Model file for the job. Use its own axes, mm. Round coordinates to 2 decimals unless told otherwise and drop trailing zeros. Loops run counter-clockwise (first coordinate to the right, second up) from the corner with the lowest first, then second, coordinate; pieces in that order, holes last. Notation, with made-up numbers: M 39,12 L 89,12 A24 ccw 89,33 Z; hole C -38.5,16 d9. An arc over 180 degrees is marked long. Use a Markdown table: item, result. Add a question column.
Q1. Pin check, flat tips, straight feed: pin 1 (5.5 mm diameter, centred on x = -31.75, y = -6.35, fed in from -Z); pin 2 (2 mm diameter, centred on x = 81.5, y = -4.5, fed in from +Z); pin 3 (6.5 mm diameter, centred on x = 82.55, y = -6.35, fed in from -Z). Stop position of each tip, or through.
Q2. Cut at A-A (z = 3.5). Give the cut face in (x, y).
Q3. Cut at D-D (x = 82.55). Give the cut face in (y, z).
Q4. Cut at B-B (x = 120.65). Give the cut face in (y, z), plus the area to 3 significant figures.
Q5. Cut at C-C (y = -6.35). State how many separate pieces and enclosed holes the cut face has, plus the area to 3 significant figures.
Q6. Probe line 1 (X direction, y = -6.35, z = 7.25); line 2 (X direction, y = -11, z = 4.5); line 3 (Y direction, x = 82.55, z = 11.5). List the from-to ranges inside material, lowest first. Write a range as from..to.
from build123d import *

# Parameters (mm, degrees)
F0_W      = 254
F0_H      = 12.7
F1_DEPTH  = 12.7
F2_W      = 12.7
F2_H      = 6.35
F3_DEPTH  = 12.701
F4_R      = 2.794
F5_DEPTH  = 6.351
F6_R      = 4.7625
F7_DEPTH  = 5.08
F8_R      = 2.794
F9_DEPTH  = 12.701
F10_R     = 4.7625
F10_R_2   = 2.794
F11_DEPTH = 5.08


with BuildPart() as f1:
    # F0 (on Top) → F1 (new body)
    with BuildSketch(Plane.XY):
        with Locations((0, -6.35)):
            Rectangle(F0_W, F0_H)
    extrude(amount=F1_DEPTH)

    # F2 (on face) → F3 (cut, through all)
    with BuildSketch(Plane.XZ.offset(12.7)):
        with Locations((82.55, 3.175)):
            Rectangle(F2_W, F2_H)
        with Locations((31.75, 3.175)):
            Rectangle(F2_W, F2_H)
        with Locations((-31.75, 3.175)):
            Rectangle(F2_W, F2_H)
        with Locations((-82.55, 3.175)):
            Rectangle(F2_W, F2_H)
    extrude(amount=-F3_DEPTH, mode=Mode.SUBTRACT)

    # F4 (on face) → F5 (cut, through all)
    with BuildSketch(Plane(origin=(0, 0, 6.35), x_dir=(1, 0, 0), z_dir=(0, 0, -1))):
        with Locations((82.55, 6.35)):
            Circle(F4_R)
        with Locations((31.75, 6.35)):
            Circle(F4_R)
        with Locations((-82.55, 6.35)):
            Circle(F4_R)
        with Locations((-31.75, 6.35)):
            Circle(F4_R)
    extrude(amount=-F5_DEPTH, mode=Mode.SUBTRACT)

    # F6 (on face) → F7 (cut)
    with BuildSketch(Plane.XY.offset(12.7)):
        with Locations((82.55, -6.35)):
            Circle(F6_R)
        with Locations((31.75, -6.35)):
            Circle(F6_R)
        with Locations((-82.55, -6.35)):
            Circle(F6_R)
        with Locations((-31.75, -6.35)):
            Circle(F6_R)
    extrude(amount=-F7_DEPTH, mode=Mode.SUBTRACT)

    # F8 (on face) → F9 (cut, through all)
    with BuildSketch(Plane(origin=(0, 0, 0), x_dir=(1, 0, 0), z_dir=(0, 0, -1))):
        with Locations((120.65, 6.35)):
            Circle(F8_R)
    extrude(amount=-F9_DEPTH, mode=Mode.SUBTRACT)

    # F10 (on face) → F11 (cut)
    with BuildSketch(Plane.XY.offset(12.7)):
        with Locations((120.65, -6.35)):
            Circle(F10_R)
        with Locations((120.65, -6.35)):
            Circle(F10_R_2, mode=Mode.SUBTRACT)
    extrude(amount=-F11_DEPTH, mode=Mode.SUBTRACT)


solid = f1.part
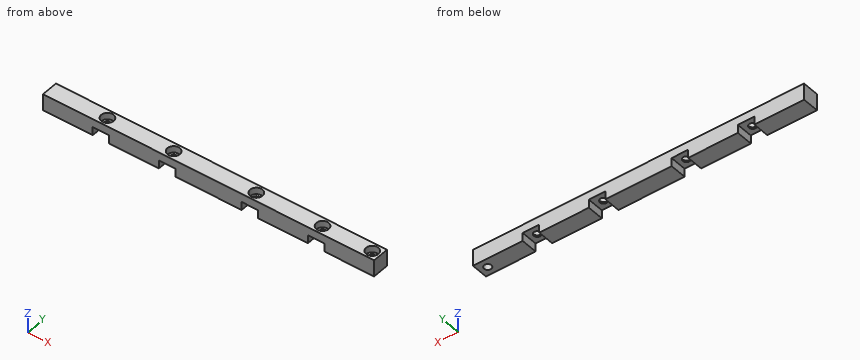
Checked values:
| question | item | result |
|---|---|---|
| 1 | pin 1 | passes through |
| 1 | pin 2 | stops at z = 7.62 |
| 1 | pin 3 | stops at z = 6.35 |
| 2 | outline | M -127,-12.7 L -88.9,-12.7 L -88.9,0 L -127,0 Z; M -76.2,-12.7 L -38.1,-12.7 L -38.1,0 L -76.2,0 Z; M -25.4,-12.7 L 25.4,-12.7 L 25.4,0 L -25.4,0 Z; M 38.1,-12.7 L 76.2,-12.7 L 76.2,0 L 38.1,0 Z; M 88.9,-12.7 L 127,-12.7 L 127,0 L 88.9,0 Z; hole C 120.65,-6.35 d5.59 |
| 3 | outline | M -12.7,6.35 L -9.14,6.35 L -9.14,7.62 L -11.11,7.62 L -11.11,12.7 L -12.7,12.7 Z; M -3.56,6.35 L 0,6.35 L 0,12.7 L -1.59,12.7 L -1.59,7.62 L -3.56,7.62 Z |
| 4 | outline | M -12.7,0 L -9.14,0 L -9.14,7.62 L -11.11,7.62 L -11.11,12.7 L -12.7,12.7 Z; M -3.56,0 L 0,0 L 0,12.7 L -1.59,12.7 L -1.59,7.62 L -3.56,7.62 Z |
| 4 | area | 70.3 mm^2 |
| 5 | separate pieces | 6 |
| 5 | enclosed holes | 0 |
| 5 | area | 2,590 mm^2 |
| 6 | line 1 | x = -127..-85.34, -79.76..-34.54, -28.96..28.96, 34.54..79.76, 85.34..117.86, 123.44..127 |
| 6 | line 2 | x = -127..-88.9, -76.2..-38.1, -25.4..25.4, 38.1..76.2, 88.9..127 |
| 6 | line 3 | y = -12.7..-11.11, -1.59..0 |
